The listing builds one solid part. Answer for the finished solid, in the listing's coordinates (mm). A direction names the side the tool comes from. Coordinates: 2 decimals unless noted, no trailing zeros. Order: outer loops, then holes, each group sorted by start corner. A loop starts at its lowest first (then second) coordinate and runs counter-clockwise, first axis right, second up.
from build123d import *

# Parameters (mm, degrees)
SKETCH1_R           = 0.45
SKETCH1_R_2         = 0.6
BOSS_EXTRUDE1_DEPTH = 3
SKETCH1_22_R        = 0.996628177
SKETCH1_22_R_2      = 0.45
BOSS_EXTRUDE2_DEPTH = 8


with BuildPart() as part:
    # Sketch1 → Boss-Extrude1 (new body)
    with BuildSketch(Plane(origin=(0, 0, 0), x_dir=(1, 0, 0), z_dir=(0, 1, 0))):
        with BuildLine():
            ThreePointArc((0.1641009, 1.993256355), (0.024548565, 1.994973575), (-0.113883759, 1.977245221))
            Line((-0.113883759, 1.977245221), (-4.183235691, 1.164159973))
            ThreePointArc((-4.183235691, 1.164159973), (-4.514100231, 1.033532975), (-4.77830642, 0.795352694))
            ThreePointArc((-4.77830642, 0.795352694), (-5.05, 0), (-4.77830642, -0.795352694))
            ThreePointArc((-4.77830642, -0.795352694), (-4.514100231, -1.033532975), (-4.183235691, -1.164159973))
            Line((-4.183235691, -1.164159973), (-0.11388376, -1.977245221))
            ThreePointArc((-0.11388376, -1.977245221), (0.024548564, -1.994973575), (0.164100898, -1.993256355))
            ThreePointArc((0.164100898, -1.993256355), (2, -1e-09), (0.1641009, 1.993256355))
        make_face()
        with Locations(Location((-3, 0, 0), (0, 0, 270))):
            Circle(SKETCH1_R, mode=Mode.SUBTRACT)
        with Locations(Location((-1.25, 0, 0), (0, 0, 270))):
            Circle(SKETCH1_R_2, mode=Mode.SUBTRACT)
        with Locations(Location((0.5, 0, 0), (0, 0, 270))):
            Circle(SKETCH1_R, mode=Mode.SUBTRACT)
    extrude(amount=BOSS_EXTRUDE1_DEPTH)

    # Sketch1_22 → Boss-Extrude2 (add)
    with BuildSketch(Plane(origin=(0, 0, 0), x_dir=(1, 0, 0), z_dir=(0, 1, 0))):
        with Locations(Location((0.5, 0, 0), (0, 0, 270))):
            Circle(SKETCH1_22_R)
        with Locations(Location((0.5, 0, 0), (0, 0, 270))):
            Circle(SKETCH1_22_R_2, mode=Mode.SUBTRACT)
    extrude(amount=BOSS_EXTRUDE2_DEPTH)


solid = part.part
1) Each of these flat-tipped pins is pushed along its axis until it touches: P1, Ø4, axis at x = 0, y = 6, coming from the +Z side; P2, Ø1.5, axis at y = 6, z = 1, coming from the +X side; P3, Ø1, axis at x = -1.25, z = 0, coming from the +Y side (1 decimal); P4, Ø1.5, axis at x = 1, y = 3.5, coming from the +Z side. Where does it stop, or does it pass through?
2) Section B-B (x = -1.25) is taken. Give the vertices of the cut face in (y, z).
3) Determine the mould class of faces 3 (the face through (2, 1, 0)), 4 (the face through (-3.44, 1.48, -0.1)), 5 (the face through (-2, 0, 1)) for opening direction Z: released by +Z, released by -Z, zero draft, split by the parting line, or undercut.
4) Section C-C (y = 1) is taken. Give the vertices of the cut face in (x, z).
5) Consider L1, parallel to Y at x = -2, z = -1.2; L2, parallel to X at y = 4.5, z = 0; L3, parallel to Z at x = 0, y = 2. Determine where each line is inside the solid, lowest interval first.
6) Section A-A (z = 0) is taken. Give the vertices of the cut face in (x, y), then the cut area to 3 significant figures.
7) Section D-D (y = 4) is taken. Give the vertices of the cut face in (x, z).
8) A tool of negligible diameter and unlimited length cuts with its end or side. For faces 1 (the face through (-0.47, 5.46, -0.22)), 2 (the face through (-5.05, 1.48, -0.01)), from which of +Z, -Z, +X, -X, +Y, -Y can it reach the whole face along a straight path? Write none if from no direction.
Filled sheet:
1. P1: stops at z = 1
1. P2: stops at x = 1.46
1. P3: passes through
1. P4: stops at z = 1.95
2. outline: (0, -1.75) - (3, -1.75) - (3, -0.6) - (0, -0.6) - close; (0, 0.6) - (3, 0.6) - (3, 1.75) - (0, 1.75) - close
3. face 3: split by the parting line
3. face 4: undercut
3. face 5: zero draft
4. outline: (-4.78, -0.8) arc R1 ccw to (-4.18, -1.16) - (-0.11, -1.98) arc R1 ccw to (0.16, -1.99) arc R2 ccw to (0.16, 1.99) arc R1 ccw to (-0.11, 1.98) - (-4.18, 1.16) arc R1 ccw to (-4.78, 0.8) arc R1.3 ccw to start; hole circle Ø0.9 at (-3, 0); hole circle Ø1.2 at (-1.25, 0); hole circle Ø0.9 at (0.5, 0)
5. L1: y = 0 to 3
5. L2: x = -0.5 to 0.05, 0.95 to 1.5
5. L3: z = -1.99 to 1.99
6. outline: (-5.05, 0) - (-3.45, 0) - (-3.45, 3) - (-5.05, 3) - close; (-2.55, 0) - (-1.85, 0) - (-1.85, 3) - (-2.55, 3) - close; (-0.65, 0) - (0.05, 0) - (0.05, 8) - (-0.5, 8) - (-0.5, 3) - (-0.65, 3) - close; (0.95, 0) - (2, 0) - (2, 3) - (1.5, 3) - (1.5, 8) - (0.95, 8) - close
6. area: 17.6 mm2
7. outline: circle Ø1.99 at (0.5, 0); hole circle Ø0.9 at (0.5, 0)
8. face 1: +Y
8. face 2: -X, +Y, -Y
